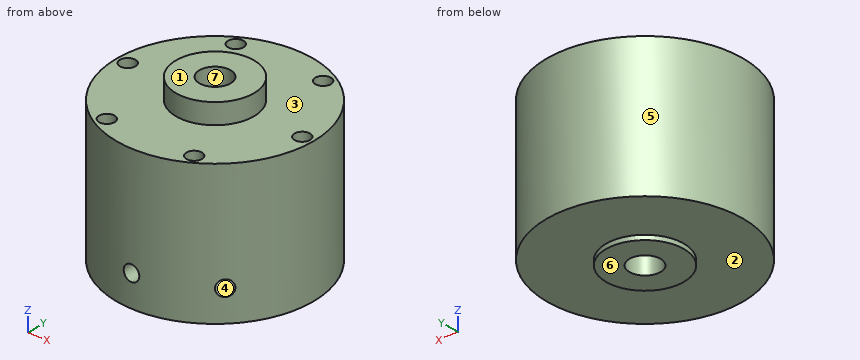
from build123d import *

# Parameters (mm, degrees)
SKETCH_2_R          = 12.5
EXTRUDE_1_DEPTH     = 1.5
SKETCH_3_R          = 31.5
EXTRUDE_2_DEPTH     = 45
SKETCH_4_R          = 12.5
EXTRUDE_3_DEPTH     = 6.5
SKETCH_5_R          = 5
CUT_EXTRUDE_1_DEPTH = 70.235106702
SKETCH_6_R          = 2.5
CUT_EXTRUDE_2_DEPTH = 70.235106702
SKETCH_7_R          = 2.5
CUT_EXTRUDE_3_DEPTH = 70.235106869
SKETCH_8_R          = 2.5
CUT_EXTRUDE_4_DEPTH = 10
SKETCH_9_R          = 2.5
CUT_EXTRUDE_5_DEPTH = 16


with BuildPart() as part:
    # 草图2 → 凸台-拉伸1 (new body)
    with BuildSketch(Plane.XY):
        Circle(SKETCH_2_R)
    extrude(amount=EXTRUDE_1_DEPTH)

    # 草图3 → 凸台-拉伸2 (add)
    with BuildSketch(Plane.XY.offset(1.5)):
        with Locations(Location((0, 0, 0), (0, 0, 180))):
            Circle(SKETCH_3_R)
    extrude(amount=EXTRUDE_2_DEPTH)

    # 草图4 → 凸台-拉伸3 (add)
    with BuildSketch(Plane.XY.offset(46.5)):
        Circle(SKETCH_4_R)
    extrude(amount=EXTRUDE_3_DEPTH)

    # 草图5 → 切除-拉伸1 (cut, through all)
    with BuildSketch(Plane.XY.offset(53)):
        Circle(SKETCH_5_R)
    extrude(amount=-CUT_EXTRUDE_1_DEPTH, mode=Mode.SUBTRACT)

    # 草图6 → 切除-拉伸2 (cut, through all)
    with BuildSketch(Plane(origin=(0, 0, 0), x_dir=(0.7071067811865477, 0.7071067811865475, 0), z_dir=(-0.7071067811865475, 0.7071067811865477, 0))):
        with Locations(Location((0, -11.5, 0), (0, 0, 180))):
            Circle(SKETCH_6_R)
    extrude(amount=-CUT_EXTRUDE_2_DEPTH, mode=Mode.SUBTRACT)

    # 草图7 → 切除-拉伸3 (cut, through all)
    with BuildSketch(Plane(origin=(0, 0, 0), x_dir=(1, 0, 0), z_dir=(0, 1, 0))):
        with Locations(Location((0, -11.5, 0), (0, 0, 270))):
            Circle(SKETCH_7_R)
    extrude(amount=-CUT_EXTRUDE_3_DEPTH, mode=Mode.SUBTRACT)

    # 草图8 → 切除-拉伸4 (cut)
    with BuildSketch(Plane.XY.offset(46.5)):
        with Locations((28, 0)):
            Circle(SKETCH_8_R)
        with Locations((-14, -24.248711306)):
            Circle(SKETCH_8_R)
        with Locations((-14, 24.248711306)):
            Circle(SKETCH_8_R)
    extrude(amount=-CUT_EXTRUDE_4_DEPTH, mode=Mode.SUBTRACT)

    # 草图9 → 切除-拉伸5 (cut)
    with BuildSketch(Plane.XY.offset(46.5)):
        with Locations((-28, 0)):
            Circle(SKETCH_9_R)
        with Locations((14, 24.248711306)):
            Circle(SKETCH_9_R)
        with Locations((14, -24.248711306)):
            Circle(SKETCH_9_R)
    extrude(amount=-CUT_EXTRUDE_5_DEPTH, mode=Mode.SUBTRACT)


solid = part.part
Geometry: final body of the model. Coordinates: model frame, mm. Face numbers are marked on the shaded views. A direction names the side the tool comes from. Coordinates: 2 decimals unless noted, no trailing zeros. Loops run counter-clockwise (first coordinate to the right, second up) from the corner with the lowest first, then second, coordinate; pieces in that order, holes last. Notation, with made-up numbers: (-34.75, 87) - (15.25, 87) arc R21 ccw to (15.25, 92) - close; hole circle Ø11 at (0.5, -29). An arc over 180 degrees is marked (long way). Put each result on its own line as item: value. Start each with the question number.
Q1. Cut plane D-D, the plane z = 31.5. Return loops of the section in (x, y).
Q2. Pull-direction query (Y, two-part tool) for the marked faces 4, 5, 6 and 7; classes: released by +Y, released by -Y, zero draft, split by the parting line, or undercut.
Q3. Pin query (flat end, axial travel): pin 1 Ø6.5 at (x, z) = (0, 11.5) entering from +Y; pin 2 Ø4 at (y, z) = (-12.5, 25) entering from +X; pin 3 Ø6 at (x, y) = (0, 0) entering from -Z; pin 4 Ø1 at (x, y) = (5.5, 12.5) entering from +Z. Return the tip coordinate at first contact, or that it passes through.
Q4. Set-up query: the marked faces 1, 2 and 3. Return all of +Z, -Z, +X, -X, +Y, -Y with unobstructed straight access to the full face (end or side cutting, diameter ignored); none if empty.
Q5. Cut plane A-A, the plane y = 0. Return loops of the section in (x, z), and give its area (4 significant figures).
Q6. Line query: line 1 (Y direction, x = 0, z = 21); line 2 (Z direction, x = -6.5, y = -15); line 3 (Y direction, x = 14, z = 34). Output: solid intervals per line, ascending.
Q7. Cut plane C-C, the plane z = 48.5. Return loops of the section in (x, y).
Q8. Cut plane B-B, the plane x = 0. Return loops of the section in (y, z), and give its area (3 significant figures).
Filled sheet:
1. outline: circle Ø63 at (0, 0); hole circle Ø5 at (-28, 0); hole circle Ø10 at (0, 0); hole circle Ø5 at (14, -24.25); hole circle Ø5 at (14, 24.25)
2. face 4: undercut
2. face 5: split by the parting line
2. face 6: zero draft
2. face 7: undercut
3. pin 1: y = 31.5
3. pin 2: x = 29.7
3. pin 3: through
3. pin 4: z = 46.5
4. face 1: +Z, +X, -X, +Y, -Y
4. face 2: -Z
4. face 3: +Z
5. outline: (-31.5, 1.5) - (-12.5, 1.5) - (-12.5, 0) - (-5, 0) - (-5, 53) - (-12.5, 53) - (-12.5, 46.5) - (-25.5, 46.5) - (-25.5, 30.5) - (-30.5, 30.5) - (-30.5, 46.5) - (-31.5, 46.5) - close; (5, 0) - (12.5, 0) - (12.5, 1.5) - (31.5, 1.5) - (31.5, 46.5) - (30.5, 46.5) - (30.5, 36.5) - (25.5, 36.5) - (25.5, 46.5) - (12.5, 46.5) - (12.5, 53) - (5, 53) - close
5. area: 2,375 mm²
6. line 1: -31.5 to -5, 5 to 31.5
6. line 2: 1.5 to 46.5
6. line 3: -28.22 to -26.75, -21.75 to 21.75, 26.75 to 28.22
7. outline: circle Ø25 at (0, 0); hole circle Ø10 at (0, 0)
8. outline: (-31.5, 1.5) - (-12.5, 1.5) - (-12.5, 0) - (-5, 0) - (-5, 9) - (-31.5, 9) - close; (-31.5, 14) - (-5, 14) - (-5, 53) - (-12.5, 53) - (-12.5, 46.5) - (-31.5, 46.5) - close; (5, 0) - (12.5, 0) - (12.5, 1.5) - (31.5, 1.5) - (31.5, 46.5) - (12.5, 46.5) - (12.5, 53) - (5, 53) - close
8. area: 2,370 mm²
